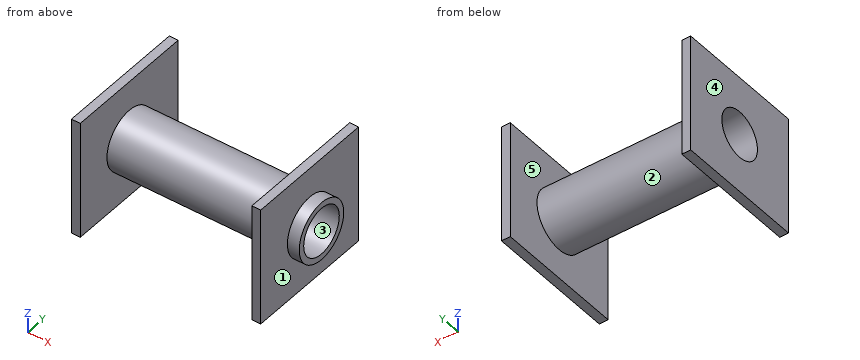
Autodesk Inventor part; units mm, degrees
ref_plane "YZ Plane" through (0, 0, 0) normal (1, 0, 0) x (0, 1, 0)
ref_plane "XZ Plane" through (0, 0, 0) normal (0, 1, 0) x (-1, 0, 0)
ref_plane "XY Plane" through (0, 0, 0) normal (0, 0, 1) x (1, 0, 0)
sketch "Эскиз1" plane through (0, 0, 0) normal (1, 0, 0) x (0, 1, 0)
  line L0 (-11, 10) -> (11, 10)
  line L1 (11, 10) -> (11, -10)
  line L2 (11, -10) -> (-11, -10)
  line L3 (-11, -10) -> (-11, 10)
  line L4 (-11, 10) -> (11, -10) construction
  line L5 (11, 10) -> (-11, -10) construction
  circle A0 centre (0, 0) radius 5
  dimension "d1" = 22
  dimension "d2" = 20
  dimension "d3" = 10
extrude "Выдавливание1" add sketch "Эскиз1" along normal blind 1.5
ref_plane "РабПлоскость1" through (16, 0, 0) normal (1, 0, 0) x (0, 0, -1)
mirror "Зеркальное отражение1" about plane through (16, 0, 0) normal (1, 0, 0) of "Выдавливание1"
sketch "Эскиз2" plane through (0, 0, 0) normal (-1, 0, 0) x (0, 0, 1)
  circle A0 centre (0, 0) radius 5
  circle A1 centre (0, 0) radius 4
  dimension "d7" = 8
extrude "Выдавливание2" add sketch "Эскиз2" against normal blind 34
properties part number "frame" material "Пластмасса, непрозрачная, черная"
Verification items for the finished model (mm, model axes). Face numbers are marked on the shaded views. A direction names the side the tool comes from. Give positions to 0.01 mm unless a question says otherwise; leave off trailing zeros. Order: outer loops, then holes, each group sorted by start corner. A loop starts at its lowest first (then second) coordinate and runs counter-clockwise, first axis right, second up. Notation, with made-up numbers: M 71,72 L 84,72 A32 ccw 84,101 Z; hole C -18.5,31 d6. An arc over 180 degrees is marked long. Use one line per item in the form item = value. Start each with the question number.
Q1. Section check A-A (y = 0). Enter the section's corners in (x, z).
Q2. Section check C-C (x = 11). Enter the section's corners in (y, z), then the cut area to 3 significant figures.
Q3. Section check B-B (z = 0). Enter the section's corners in (x, y).
Q4. Go/stop test with flat-tipped pins: pin 1 Ø1.5 at (x, y) = (3.5, 4.5) entering from +Z; pin 2 Ø5 at (x, y) = (27, 5) entering from +Z; pin 3 Ø5 at (x, y) = (14.5, 6) entering from -Z; pin 4 Ø7 at (y, z) = (0, 0) entering from -X. Record where each tip stops, or that it passes through.
Q5. Access from +Z, -Z, +X, -X, +Y, -Y to the whole of each face (thin tool, end or side, straight path). Record for the marked faces 4 and 5.
Q6. Section check D-D (y = -6.25). Enter the section's corners in (x, z), then the cut area to 3 significant figures.
Q7. Mould release check, pull along Z, two halves, no side actions. Record for the marked faces 1, 2 and 3: +Z half, -Z half, draft (parallel to the pull), parting line (faces both ways), or undercut.
Q8. Scan lines: line 1 along X through (y, z) = (3.25, -4.75); line 2 along Y through (x, z) = (31.5, 0.25); line 3 along Z through (x, y) = (32.5, 0.25). Record each from-to range of solid material in increasing order. Write a range as [from, to].
Evaluation:
q1.outline = M 0,-10 L 1.5,-10 L 1.5,-5 L 30.5,-5 L 30.5,-10 L 32,-10 L 32,-5 L 34,-5 L 34,-4 L 0,-4 Z; M 0,4 L 34,4 L 34,5 L 32,5 L 32,10 L 30.5,10 L 30.5,5 L 1.5,5 L 1.5,10 L 0,10 Z
q2.outline = C 0,0 d10; hole C 0,0 d8
q2.area = 28.3 mm2
q3.outline = M 0,-11 L 1.5,-11 L 1.5,-5 L 30.5,-5 L 30.5,-11 L 32,-11 L 32,-5 L 34,-5 L 34,-4 L 0,-4 Z; M 0,4 L 34,4 L 34,5 L 32,5 L 32,11 L 30.5,11 L 30.5,5 L 1.5,5 L 1.5,11 L 0,11 Z
q4.pin_1 = 3.31
q4.pin_2 = 4.33
q4.pin_3 = -3.57
q4.pin_4 = through
q5.face_4 = +Z, -Z, -X, +Y, -Y
q5.face_5 = none
q6.outline = M 0,-10 L 1.5,-10 L 1.5,10 L 0,10 Z; M 30.5,-10 L 32,-10 L 32,10 L 30.5,10 Z
q6.area = 60.0 mm2
q7.face_1 = draft
q7.face_2 = parting line
q7.face_3 = undercut
q8.line_1 = [0, 1.5], [30.5, 32]
q8.line_2 = [-11, -3.99], [3.99, 11]
q8.line_3 = [-4.99, -3.99], [3.99, 4.99]
